Source: three-view drawing plus pictorial views. Frame: mm from the lowest corner of the part. A direction names the side the tool comes from. Coordinates: 2 decimals unless noted, no trailing zeros. Order: outer loops, then holes, each group sorted by start corner. A loop starts at its lowest first (then second) coordinate and runs counter-clockwise, first axis right, second up. Notation, with made-up numbers: (71.5, 12.5) -> (101.5, 12.5) arc R31 cw to (101.5, 48.5) -> close; hole circle Ø2 at (40, -34). An arc over 180 degrees is marked (long way). One line per question, with ' | ' between items.
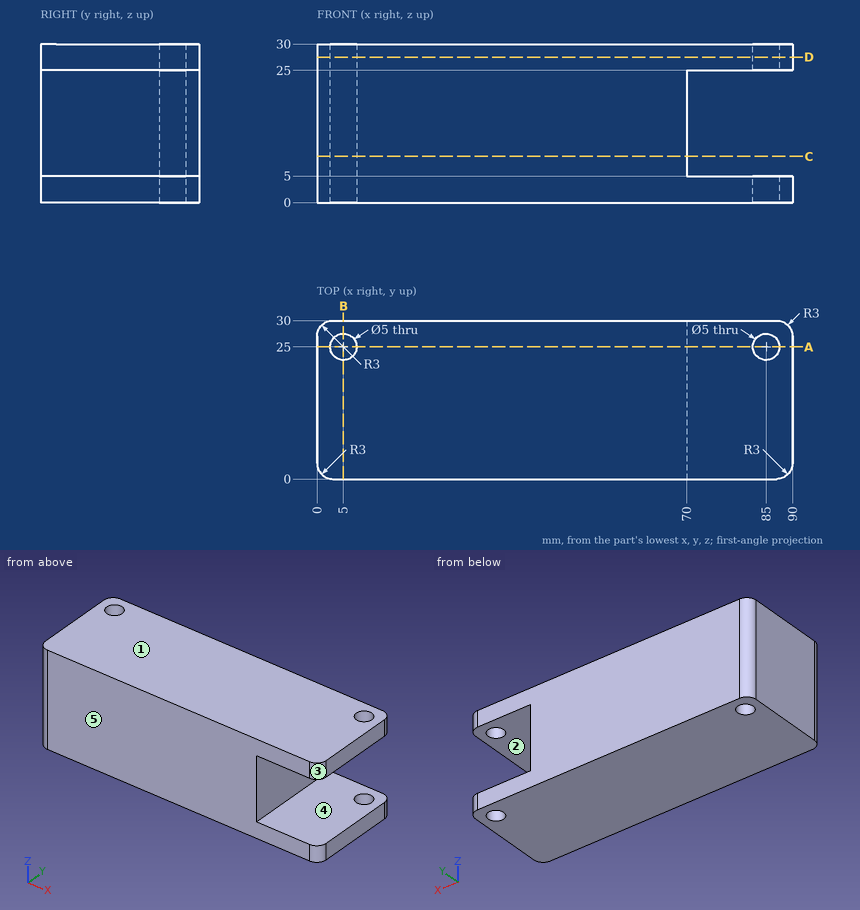
1. Cut plane C-C, the plane z = 8.75. Return loops of the section in (x, y).
Recorded:
outline: (0, 3) arc R3 ccw to (3, 0) -> (70, 0) -> (70, 30) -> (3, 30) arc R3 ccw to (0, 27) -> close; hole circle Ø5 at (5, 25)
2. Cut plane A-A, the plane y = 25. Return loops of the section in (x, z), and give its area (3 significant figures).
Recorded:
outline: (0, 0) -> (2.5, 0) -> (2.5, 30) -> (0, 30) -> close; (7.5, 0) -> (82.5, 0) -> (82.5, 5) -> (70, 5) -> (70, 25) -> (82.5, 25) -> (82.5, 30) -> (7.5, 30) -> close; (87.5, 0) -> (90, 0) -> (90, 5) -> (87.5, 5) -> close; (87.5, 25) -> (90, 25) -> (90, 30) -> (87.5, 30) -> close | area: 2,100 mm^2
3. Cut plane D-D, the plane z = 27.5. Return loops of the section in (x, y), and give its area (3 significant figures).
Recorded:
outline: (0, 3) arc R3 ccw to (3, 0) -> (87, 0) arc R3 ccw to (90, 3) -> (90, 27) arc R3 ccw to (87, 30) -> (3, 30) arc R3 ccw to (0, 27) -> close; hole circle Ø5 at (5, 25); hole circle Ø5 at (85, 25) | area: 2,650 mm^2
4. Cut plane B-B, the plane x = 5. Return loops of the section in (y, z), and give its area (3 significant figures).
Recorded:
outline: (0, 0) -> (22.5, 0) -> (22.5, 30) -> (0, 30) -> close; (27.5, 0) -> (30, 0) -> (30, 30) -> (27.5, 30) -> close | area: 750 mm^2
5. Access query for the marked faces 4 and 5. Directions: +Z, -Z, +X, -X, +Y, -Y. A direction counts if a zero-diameter tool reaches every point of the face in a straight line with its end or side. Return the directions, or none.
Recorded:
face 4: +X, +Y, -Y | face 5: +Z, -Z, +X, -X, -Y
6. Pin query (flat end, axial travel): pin 1 Ø4 at (x, y) = (5, 25) entering from -Z; pin 2 Ø4 at (y, z) = (6, 14) entering from +X. Return the tip coordinate at first contact, or that it passes through.
Recorded:
pin 1: passes through | pin 2: stops at x = 70
7. Ray query, line 1 (Z direction, x = 79, y = 25.25); line 2 (Y direction, x = 85, z = 26.6); line 3 (X direction, y = 20.75, z = 6.5). Return the intervals inside material, ascending. Write a range as [from, to].
Recorded:
line 1: z = [0, 5], [25, 30] | line 2: y = [0, 22.5], [27.5, 30] | line 3: x = [0, 70]
8. Mould query, pull axis Z, two halves, no side actions, for the marked faces 1, 2 and 3. Classes: released by +Z, released by -Z, zero draft, split by the parting line, or undercut.
Recorded:
face 1: released by +Z | face 2: undercut | face 3: zero draft
